For this review, take the finished solid that the model builds, in its own axes (mm). Face numbers are marked on the shaded views. A direction names the side the tool comes from. Coordinates: 2 decimals unless noted, no trailing zeros. Order: outer loops, then holes, each group sorted by start corner. A loop starts at its lowest first (then second) coordinate and runs counter-clockwise, first axis right, second up. Notation, with made-up numbers: (13.25, -21.75) -> (62.25, -21.75) arc R37 ccw to (62.25, 16.25) -> close; hole circle Ø8 at (0.5, -20). An arc over 180 degrees is marked (long way). Return JSON: item names as keys, results as strings. Group by question number.
Item 1: Take a section at C-C (z = 1.8). Write out the cut boundary in (x, y), then the cut area to 3 significant figures.
Item 2: Insertion check: pin 1 (0.9 mm diameter, centred on x = -0.5, y = -0.5, fed in from -Z); pin 2 (1 mm diameter, centred on x = 1, y = -1, fed in from +Z); pin 3 (1.4 mm diameter, centred on y = -1.5, z = 0, fed in from +X). Each pin has a flat end and moves straight along its axis. Give the tip position at first contact, or say it passes through.
Item 3: Take a section at B-B (x = -1). Write out the cut boundary in (y, z).
Item 4: Take a section at D-D (x = 2.25). Write out the cut boundary in (y, z), then the cut area to 3 significant figures.
Item 5: For line 1 along Y through (x, z) = (2.25, -0.6), list the stretches that pass through material, from the lowest coordinate up.
Item 6: Machinability: for the marked faces 1, 2, 3, 4 and 5, which of the approach directions +Z, -Z, +X, -X, +Y, -Y give a long, thin tool a straight path to every point of the face, cutting with its end or side? Answer none if there is none.
Item 7: Take a section at A-A (z = 0.45). Write out the cut boundary in (x, y).
```python
from build123d import *

# Parameters (mm, degrees)
F0_W     = 7.7
F0_H     = 4.3
F0_W_2   = 3
F0_H_2   = 1.5
F1_DEPTH = 4.3
F2_DEPTH = 2
F3_R     = 0.2
F4_R     = 0.1


with BuildPart() as f1:
    # F0 (on Front) → F1 (new body)
    with BuildSketch(Plane.XZ):
        Rectangle(F0_W, F0_H)
        Rectangle(F0_W_2, F0_H_2, mode=Mode.SUBTRACT)
        Rectangle(F0_W_2, F0_H_2)
    extrude(amount=-F1_DEPTH)

    # F0 (on Front) → F2 (join)
    with BuildSketch(Plane.XZ):
        Rectangle(F0_W_2, F0_H_2)
    extrude(amount=F2_DEPTH)

    # F3
    f3_edges = [f1.edges().sort_by_distance(p)[0] for p in [
        (0, -2, 0.75),
        (1.5, -2, 0),
        (0, -2, -0.75),
        (-1.5, -2, 0),
    ]]
    fillet(f3_edges, radius=F3_R)

    # F4
    f4_edges = [f1.edges().sort_by_distance(p)[0] for p in [
        (1.42921, -1.952659, 0.67921),
        (1.42921, -1.952659, -0.67921),
        (-1.42921, -1.952659, -0.67921),
        (-1.42921, -1.952659, 0.67921),
    ]]
    fillet(f4_edges, radius=F4_R)


solid = f1.part
```
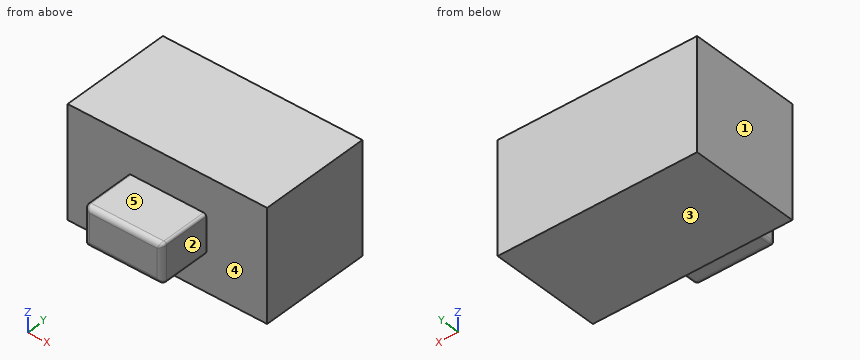
Findings below:
{
 "1": {"outline": "(-3.85, 0) -> (3.85, 0) -> (3.85, 4.3) -> (-3.85, 4.3) -> close", "area": "33.1 mm2"},
 "2": {"pin 1": "stops at z = -0.75", "pin 2": "stops at z = 0.75", "pin 3": "stops at x = 1.5"},
 "3": {"outline": "(-2, -0.55) arc R0.2 ccw to (-1.8, -0.75) -> (0, -0.75) -> (0, -2.15) -> (4.3, -2.15) -> (4.3, 2.15) -> (0, 2.15) -> (0, 0.75) -> (-1.8, 0.75) arc R0.2 ccw to (-2, 0.55) -> close"},
 "4": {"outline": "(0, -2.15) -> (4.3, -2.15) -> (4.3, 2.15) -> (0, 2.15) -> close", "area": "18.5 mm2"},
 "5": {"line 1": "y = 0 to 4.3"},
 "6": {"face 1": "+Z, -Z, -X, +Y, -Y", "face 2": "+Z, -Z, +X, -Y", "face 3": "-Z, +X, -X, +Y, -Y", "face 4": "-Y", "face 5": "+Z, +X, -X, -Y"},
 "7": {"outline": "(-3.85, 0) -> (-1.5, 0) -> (-1.5, -1.8) arc R0.2 ccw to (-1.3, -2) -> (1.3, -2) arc R0.2 ccw to (1.5, -1.8) -> (1.5, 0) -> (3.85, 0) -> (3.85, 4.3) -> (-3.85, 4.3) -> close"}
}
